from build123d import *

# Parameters (mm, degrees)
SKETCH1_R           = 25
BOSS_EXTRUDE1_DEPTH = 40
SKETCH2_R           = 1.5
BOSS_EXTRUDE2_DEPTH = 15
SKETCH3_W           = 10
SKETCH3_H           = 11.292423953
BOSS_EXTRUDE3_DEPTH = 5
SKETCH4_W           = 9.492423953
SKETCH4_H           = 3.2
SKETCH4_R           = 0.75
CUT_EXTRUDE1_DEPTH  = 4


with BuildPart() as part:
    # Sketch1 → Boss-Extrude1 (new body)
    with BuildSketch(Plane(origin=(0, 0, 0), x_dir=(1, 0, 0), z_dir=(0, 1, 0))):
        Circle(SKETCH1_R)
    extrude(amount=BOSS_EXTRUDE1_DEPTH)

    # Sketch2 → Boss-Extrude2 (add)
    with BuildSketch(Plane(origin=(0, 40, 0), x_dir=(1, 0, 0), z_dir=(0, 1, 0))):
        Circle(SKETCH2_R)
    extrude(amount=BOSS_EXTRUDE2_DEPTH)

    # Sketch3 → Boss-Extrude3 (add)
    with BuildSketch(Plane.XZ):
        with Locations((24.932644211, 1.833917291)):
            Rectangle(SKETCH3_W, SKETCH3_H)
    extrude(amount=-BOSS_EXTRUDE3_DEPTH)

    # Sketch4 → Cut-Extrude1 (cut)
    with BuildSketch(Plane(origin=(29.932644211, 0, 0), x_dir=(0, 0, -1), z_dir=(1, 0, 0))):
        with Locations((-1.833917291, 2.5)):
            Rectangle(SKETCH4_W, SKETCH4_H)
        with Locations((-4.657023279, 2.5)):
            Circle(SKETCH4_R, mode=Mode.SUBTRACT)
        with Locations((0.989188698, 2.5)):
            Circle(SKETCH4_R, mode=Mode.SUBTRACT)
    extrude(amount=-CUT_EXTRUDE1_DEPTH, mode=Mode.SUBTRACT)


solid = part.part
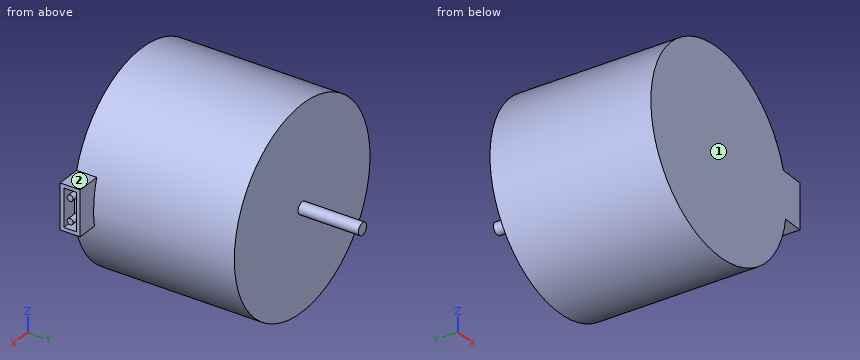
Model file for the job. Use its own axes, mm. Face numbers are marked on the shaded views. A direction names the side the tool comes from. Give positions to 0.01 mm unless a question says otherwise; leave off trailing zeros. Order: outer loops, then holes, each group sorted by start corner. A loop starts at its lowest first (then second) coordinate and runs counter-clockwise, first axis right, second up. Notation, with made-up numbers: (71, 74) -> (101, 74) arc R22 ccw to (101, 105) -> close; hole circle Ø4 at (-0.75, 75). An arc over 180 degrees is marked (long way). Use CSV: the item, a comma, the result in double quotes.
1. Band-saw the part on B-B, the plane x = 0. Give the cut face in (y, z), then the cut area to 4 significant figures.
Outcome:
outline,"(0, -25) -> (40, -25) -> (40, -1.5) -> (55, -1.5) -> (55, 1.5) -> (40, 1.5) -> (40, 25) -> (0, 25) -> close"
area,"2,045 mm²"
2. Band-saw the part on A-A, the plane y = 2.5. Give the cut face in (x, z).
Outcome:
outline,"(23.85, 7.48) arc R25 ccw (long way) to (24.71, -3.81) -> (29.93, -3.81) -> (29.93, -2.91) -> (25.93, -2.91) -> (25.93, -1.74) -> (29.93, -1.74) -> (29.93, -0.24) -> (25.93, -0.24) -> (25.93, 3.91) -> (29.93, 3.91) -> (29.93, 5.41) -> (25.93, 5.41) -> (25.93, 6.58) -> (29.93, 6.58) -> (29.93, 7.48) -> close"
3. Band-saw the part on C-C, the plane z = -14.5. Give the cut face in (x, y).
Outcome:
outline,"(-20.37, 0) -> (20.37, 0) -> (20.37, 40) -> (-20.37, 40) -> close"
4. Drop flat-ended pins along their axis: pin 1 (3.5 mm diameter, centred on x = 27.5, y = 2, fed in from +Z); pin 2 (4 mm diameter, centred on y = 6.5, z = 17, fed in from -X); pin 3 (1 mm diameter, centred on x = 15, y = 14, fed in from -Z). Give the stop position or say it passes through.
Outcome:
pin 1,"z = 7.48"
pin 2,"x = -20"
pin 3,"z = -20.37"
5. 3-axis set-ups, long thin cutter, end or side, ignore diameter. For the marked faces 1 and 2: which of +Z, -Z, +X, -X, +Y, -Y reach the whole face in a straight line?
Outcome:
face 1,"+Z, -Z, +X, -X, -Y"
face 2,"+Z, +X, +Y, -Y"
6. Band-saw the part on D-D, the plane y = 51. Give the cut face in (x, z).
Outcome:
outline,"circle Ø3 at (0, 0)"
7. Drill centre lines: line 1 along Y through (x, z) = (-4, 18.5); line 2 along X through (y, z) = (4.5, -19); line 3 along Z through (x, y) = (22.5, 17.5). Where is each one in solid material? Low to high. Write a range as from..to.
Outcome:
line 1,"0..40"
line 2,"-16.25..16.25"
line 3,"-10.9..10.9"
